from build123d import *

# Parameters (mm, degrees)
F1_DEPTH = 180
F2_W     = 10.35
F2_H     = 20
F2_H_2   = 110
F3_DEPTH = 25
F4_DEPTH = 25
F5_DEPTH = 25
F6_R     = 2.49999


# Not quite as in the source:
# - a fillet or chamfer is up to 0.001 mm smaller than in the source, because OpenCascade refuses the exact size


with BuildPart() as f1:
    # F0 (on Front) → F1 (new body)
    with BuildSketch(Plane.XZ):
        with BuildLine():
            ThreePointArc((2.4901854451, 0.9063533798), (0, -2.65), (-2.4901854451, 0.9063533798))
            Line((-2.4901854451, 0.9063533798), (-7.188648549, 2.6164540964))
            ThreePointArc((-7.188648549, 2.6164540964), (-7.5337793105, 1.3284085592), (-7.65, 0))
            ThreePointArc((-7.65, 0), (-5.4093668761, -5.4093668761), (0, -7.65))
            ThreePointArc((0, -7.65), (5.4093668761, -5.4093668761), (7.65, 0))
            ThreePointArc((7.65, 0), (7.5337793105, 1.3284085592), (7.188648549, 2.6164540964))
            Line((7.188648549, 2.6164540964), (2.4901854451, 0.9063533798))
        make_face()
        with BuildLine():
            ThreePointArc((0, -7.65), (-5.4093668761, -5.4093668761), (-7.65, 0))
            Line((-7.65, 0), (-7.65, -7.65))
            Line((-7.65, -7.65), (0, -7.65))
        make_face()
        with BuildLine():
            Line((7.65, -7.65), (7.65, 0))
            ThreePointArc((7.65, 0), (5.4093668761, -5.4093668761), (0, -7.65))
            Line((0, -7.65), (7.65, -7.65))
        make_face()
        Polygon((7.65, -7.65), (0, -7.65), (-7.65, -7.65), (-20, -7.65), (-20, -10.15), (20, -10.15), (20, -7.65), align=None)
    extrude(amount=F1_DEPTH)

    # F2 (on face) → F3 (join)
    with BuildSketch(Plane.XY.offset(-7.65)):
        with Locations((14.825, -170)):
            Rectangle(F2_W, F2_H)
        with Locations((14.825, -90)):
            Rectangle(F2_W, F2_H_2)
        with Locations((14.825, -10)):
            Rectangle(F2_W, F2_H)
    extrude(amount=F3_DEPTH)

    # F4 (cut): faces of the model
    f4_faces = [f1.faces().sort_by_distance(p)[0] for p in [
        (9.65, -10, 4.85),
        (9.65, -90, 4.85),
        (9.65, -170, 4.85),
    ]]
    extrude(f4_faces, amount=F4_DEPTH, mode=Mode.SUBTRACT)

    # F5 (cut): faces of the model
    f5_faces = [f1.faces().sort_by_distance(p)[0] for p in [
        (9.65, -10, 4.85),
        (9.65, -90, 4.85),
        (9.65, -170, 4.85),
    ]]
    extrude(f5_faces, amount=-F5_DEPTH, mode=Mode.SUBTRACT)

    # F6 (radius 2.5 in the source; OpenCascade refuses exactly that, so slightly less here)
    f6_edges = [f1.edges().sort_by_distance(p)[0] for p in [
        (-20, -90, -10.15),
        (0, -180, -10.15),
        (20, -90, -10.15),
        (0, 0, -10.15),
    ]]
    fillet(f6_edges, radius=F6_R)


solid = f1.part
Design review of the part built by this model. Coordinates are the model's own, in mm. A direction names the side the tool comes from. Coordinates: 2 decimals unless noted, no trailing zeros. Loops run counter-clockwise (first coordinate to the right, second up) from the corner with the lowest first, then second, coordinate; pieces in that order, holes last. Notation, with made-up numbers: (31, 81.5) -> (74, 81.5) arc R17 cw to (74, 92.5) -> close; hole circle Ø3 at (66.25, 17.25). An arc over 180 degrees is marked (long way). Use a Markdown table: item, result. Add a question column.
Item 1: Machinability: for faces 1 (the flat face through (0, -160, -4)), 2 (the flat face through (0, -20, -4)), 3 (the flat face through (-4.81, -27.4, 1.75)), 4 (the flat face through (-7.65, -152, -4)), 5 (the flat face through (7.65, -27, -4)), which of the approach directions +Z, -Z, +X, -X, +Y, -Y give a long, thin tool a straight path to every point of the face, cutting with its end or side? Answer none if there is none.
Item 2: Wall thickness on L1, parallel to Y at x = -6, z = -7.25; L2, parallel to X at y = -23, z = -5.75; L3, parallel to Z at x = 9, y = -53.5: over which ranges is each line inside the solid? List them lowest first. Write a range as from..to.
Item 3: Clearance check with flat-ended pins moving along their axes: P1, Ø5, axis at x = 0.5, z = -5, coming from the +Y side; P2, Ø6, axis at y = -30, z = -4.5, coming from the -X side; P3, Ø3, axis at x = -5.5, y = -75, coming from the +Z side. State where each tip first meets the part, or that it passes through.
Item 4: We need section A-A, the plane z = -5.75. Write out the cut boundary in (x, y).
Item 5: The part is to be moulded in two halves that separate along X. For faces 6 (the cylindrical face through (0.07, -27.4, -2.65)), 7 (the flat face through (7.65, -152, -4)), 8 (the flat face through (0, -35, -4)), say which applies: +X half, -X half, draft (parallel to the pull), parting line (faces both ways), or undercut.
Numbers:
| question | item | result |
|---|---|---|
| 1 | face 1 | +Z, +X, -X, -Y |
| 1 | face 2 | +Z, +X, -X, +Y |
| 1 | face 3 | +Z, +Y, -Y |
| 1 | face 4 | +Z, -X, +Y, -Y |
| 1 | face 5 | +Z, +X, +Y, -Y |
| 2 | L1 | y = -160..-145, -35..-20 |
| 2 | L2 | x = -7.65..7.65 |
| 2 | L3 | z = -10.15..-7.65 |
| 3 | P1 | stops at y = -20 |
| 3 | P2 | stops at x = -7.65 |
| 3 | P3 | stops at z = -7.65 |
| 4 | outline | (-7.65, -160) -> (7.65, -160) -> (7.65, -145) -> (-7.65, -145) -> close; (-7.65, -35) -> (7.65, -35) -> (7.65, -20) -> (-7.65, -20) -> close |
| 5 | face 6 | undercut |
| 5 | face 7 | +X half |
| 5 | face 8 | draft |
